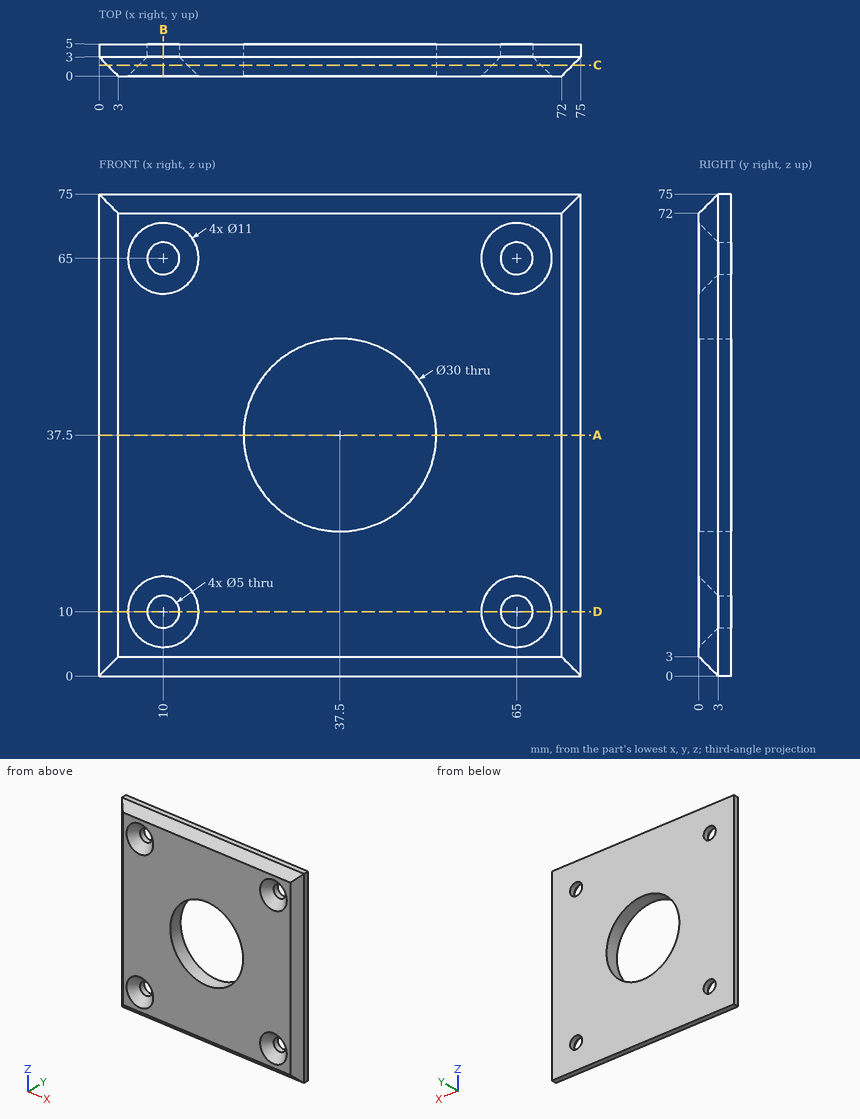
Geometry: see drawing. Coordinates: mm, zero at the bounding-box minimum. Coordinates: 2 decimals unless noted, no trailing zeros. Write each loop counter-clockwise with the first axis right and the second up, starting at its lowest first coordinate (ties: lowest second). Pieces come first, ordered by that corner, then holes.
1) Material intervals for line 1 along Z through (x, y) = (10, 3.4); line 2 along Z through (x, y) = (6, 0.9); line 3 along X through (y, z) = (4.6, 11), sorted ascending.
2) Section B-B on x = 10. Output: boundary loops of the cut face in (y, z), and give its area (3 significant figures).
3) Section C-C on y = 1.7. Output: boundary loops of the cut face in (x, z).
4) Section A-A on z = 37.5. Output: boundary loops of the cut face in (x, y).
5) Section D-D on z = 10. Output: boundary loops of the cut face in (x, y).
6) Pin query (flat end, axial travel): pin 1 Ø1 at (x, y) = (62, 1) entering from -Z; pin 2 Ø6 at (x, z) = (49, 30.5) entering from +Y; pin 3 Ø6 at (x, z) = (10, 65) entering from -Y; pin 4 Ø1 at (y, z) = (2, 55.5) entering from -X. Return the tip coordinate at first contact, or that it passes through.
Check result:
1. line 1: z = 0 to 7.5, 12.5 to 62.5, 67.5 to 75
1. line 2: z = 2.1 to 7.73, 12.27 to 62.73, 67.27 to 72.9
1. line 3: x = 0 to 7.71, 12.29 to 62.71, 67.29 to 75
2. outline: (0, 3) - (3, 0) - (5, 0) - (5, 7.5) - (3, 7.5) - (0, 4.5) - close; (0, 15.5) - (3, 12.5) - (5, 12.5) - (5, 62.5) - (3, 62.5) - (0, 59.5) - close; (0, 70.5) - (3, 67.5) - (5, 67.5) - (5, 75) - (3, 75) - (0, 72) - close
2. area: 298 mm2
3. outline: (1.3, 1.3) - (73.7, 1.3) - (73.7, 73.7) - (1.3, 73.7) - close; hole circle Ø7.6 at (10, 10); hole circle Ø7.6 at (10, 65); hole circle Ø30 at (37.5, 37.5); hole circle Ø7.6 at (65, 10); hole circle Ø7.6 at (65, 65)
4. outline: (0, 3) - (3, 0) - (22.5, 0) - (22.5, 5) - (0, 5) - close; (52.5, 0) - (72, 0) - (75, 3) - (75, 5) - (52.5, 5) - close
5. outline: (0, 3) - (3, 0) - (4.5, 0) - (7.5, 3) - (7.5, 5) - (0, 5) - close; (12.5, 3) - (15.5, 0) - (59.5, 0) - (62.5, 3) - (62.5, 5) - (12.5, 5) - close; (67.5, 3) - (70.5, 0) - (72, 0) - (75, 3) - (75, 5) - (67.5, 5) - close
6. pin 1: stops at z = 1.5
6. pin 2: stops at y = 5
6. pin 3: stops at y = 2.5
6. pin 4: stops at x = 0.5
